Input: part model. Units: mm. Frame: model coordinates. Coordinates: 2 decimals unless noted, no trailing zeros. Order: outer loops, then holes, each group sorted by start corner. A loop starts at its lowest first (then second) coordinate and runs counter-clockwise, first axis right, second up. Notation, with made-up numbers: (-26, -13) -> (29, -13) arc R11 ccw to (29, 4) -> close; hole circle Ø6 at (75, 40.5). An arc over 180 degrees is marked (long way). One line per item, written item: value. Start each with the question number.
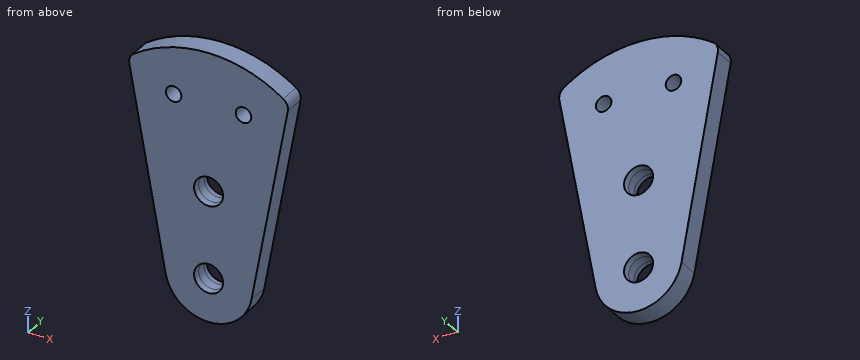
from build123d import *
from OCP.BRepFilletAPI import BRepFilletAPI_MakeChamfer

# Parameters (mm, degrees)
BOSS_EXTRUDE1_DEPTH   = 3.175
F_4_40_TAPPED_HOLE1_D = 2.2606
CUT_EXTRUDE1_REACH    = 37.03
SKETCH3_R             = 1.9812
CHAMFER1_SIZE         = 0.127
CHAMFER1_SIZE2        = 0.903651955


with BuildPart() as part:
    # Sketch2 → Boss-Extrude1 (new body)
    with BuildSketch(Plane(origin=(0, 0, 0), x_dir=(1, 0, 0), z_dir=(0, 1, 0))):
        with BuildLine():
            Line((-6.247852156, 1.134391221), (-11.522869846, -27.918663873))
            ThreePointArc((-11.522869846, -27.918663873), (-11.4270655, -28.816266687), (-10.860710811, -29.519197446))
            ThreePointArc((-10.860710811, -29.519197446), (0, -32.9184), (10.860710811, -29.519197446))
            ThreePointArc((10.860710811, -29.519197446), (11.4270655, -28.816266687), (11.522869846, -27.918663873))
            Line((11.522869846, -27.918663873), (6.247852156, 1.134391221))
            ThreePointArc((6.247852156, 1.134391221), (0, 6.35), (-6.247852156, 1.134391221))
        make_face()
    extrude(amount=BOSS_EXTRUDE1_DEPTH)

    # #4-40 Tapped Hole1 (through all)
    with Locations(Plane(origin=(0, 3.175, 0), x_dir=(1, 0, 0), z_dir=(0, 1, 0))):
        with Locations((-5.08, -25.4), (5.08, -25.4)):
            Hole(F_4_40_TAPPED_HOLE1_D / 2)

    # Sketch3 → Cut-Extrude1 (cut, up to next)
    with BuildSketch(Plane(origin=(0, 3.175, 0), x_dir=(1, 0, 0), z_dir=(0, 1, 0)), mode=Mode.PRIVATE) as cut_extrude1_sk1:
        with Locations(Location((0, 0, 0), (0, 0, 270))):
            Circle(SKETCH3_R)
    cut_extrude1_tool1 = extrude(cut_extrude1_sk1.sketch, amount=-CUT_EXTRUDE1_REACH, mode=Mode.PRIVATE) & part.part
    # Sketch3 → Cut-Extrude1 (cut, up to next)
    with BuildSketch(Plane(origin=(0, 3.175, 0), x_dir=(1, 0, 0), z_dir=(0, 1, 0)), mode=Mode.PRIVATE) as cut_extrude1_sk2:
        with Locations(Location((0, -12.7, 0), (0, 0, 270))):
            Circle(SKETCH3_R)
    cut_extrude1_tool2 = extrude(cut_extrude1_sk2.sketch, amount=-CUT_EXTRUDE1_REACH, mode=Mode.PRIVATE) & part.part
    add(cut_extrude1_tool1.solids().sort_by_distance((0, 3.175, 0))[0], mode=Mode.SUBTRACT)
    add(cut_extrude1_tool2.solids().sort_by_distance((0, 3.175, 12.7))[0], mode=Mode.SUBTRACT)

    # Chamfer1: one chamfer whose edges measure the first distance from different faces: ONE call of the kernel's chamfer builder (chamfer() names one face for all edges)
    chamfer1_edges_1 = [part.edges().sort_by_distance(p)[0] for p in [
        (0, 3.175, -1.9812),
        (0, 3.175, 10.7188),
    ]]
    chamfer1_side_1 = [part.faces().sort_by_distance(p)[0] for p in [
        (0, 3.175, 15.711859533),
    ]]
    chamfer1_edges_2 = [part.edges().sort_by_distance(p)[0] for p in [
        (0, 0, -1.9812),
        (0, 0, 10.7188),
    ]]
    chamfer1_side_2 = [part.faces().sort_by_distance(p)[0] for p in [
        (0, 0, 15.711859533),
    ]]
    chamfer1 = BRepFilletAPI_MakeChamfer(part.part.solid().wrapped)
    for e in chamfer1_edges_1:
        chamfer1.Add(CHAMFER1_SIZE, CHAMFER1_SIZE2, e.wrapped, chamfer1_side_1[0].wrapped)  # the first distance lies on this face
    for e in chamfer1_edges_2:
        chamfer1.Add(CHAMFER1_SIZE, CHAMFER1_SIZE2, e.wrapped, chamfer1_side_2[0].wrapped)  # the first distance lies on this face
    add(Compound.cast(chamfer1.Shape()), mode=Mode.REPLACE)


solid = part.part
1) Section query B-B, the plane y = 1.4. Return the cut outline in (x, z).
2) Pin query (flat end, axial travel): pin 1 Ø4 at (x, z) = (-4, 22) entering from -Y; pin 2 Ø1 at (y, z) = (1, 1) entering from -X; pin 3 Ø1 at (y, z) = (2, 20.5) entering from +X. Return the tip coordinate at first contact, or that it passes through.
3) Ray query, line 1 along Z through (x, y) = (0.75, 0.4); line 2 along X through (y, z) = (2.1, 25); line 3 along Z through (x, y) = (-1, 0.85). Return the intervals inside material, ascending. Write a range as from..to.
4) Section query D-D, the plane x = 5.08. Return the cut outline in (y, z) (3 decimals), plus the area to 3 significant figures.
5) Section query A-A, the plane x = 0. Return the cut outline in (y, z) (3 decimals).
6) Section query C-C, the plane z = 0. Return the cut outline in (x, y) (3 decimals), plus the area to 3 significant figures.
Entries:
1. outline: (-11.52, 27.92) -> (-6.25, -1.13) arc R6.35 ccw to (6.25, -1.13) -> (11.52, 27.92) arc R1.6 ccw to (10.86, 29.52) arc R19.05 ccw to (-10.86, 29.52) arc R1.6 ccw to start; hole circle Ø2.26 at (-5.08, 25.4); hole circle Ø3.96 at (0, 0); hole circle Ø3.96 at (0, 12.7); hole circle Ø2.26 at (5.08, 25.4)
2. pin 1: stops at y = 0
2. pin 2: stops at x = -6.73
2. pin 3: stops at x = 10.27
3. line 1: z = -6.31..-1.91, 1.91..10.79, 14.61..32.9
3. line 2: x = -10.99..-6.14, -4.02..4.02, 6.14..10.99
3. line 3: z = -6.27..-1.72, 1.72..10.98, 14.42..32.89
4. outline: (0, -3.81) -> (3.175, -3.81) -> (3.175, 24.27) -> (0, 24.27) -> close; (0, 26.53) -> (3.175, 26.53) -> (3.175, 32.229) -> (0, 32.229) -> close
4. area: 107 mm2
5. outline: (0, -6.35) -> (3.175, -6.35) -> (3.175, -2.108) -> (2.271, -1.981) -> (0.904, -1.981) -> (0, -2.108) -> close; (0, 2.108) -> (0.904, 1.981) -> (2.271, 1.981) -> (3.175, 2.108) -> (3.175, 10.592) -> (2.271, 10.719) -> (0.904, 10.719) -> (0, 10.592) -> close; (0, 14.808) -> (0.904, 14.681) -> (2.271, 14.681) -> (3.175, 14.808) -> (3.175, 32.918) -> (0, 32.918) -> close
6. outline: (-6.454, 0) -> (-2.108, 0) -> (-1.981, 0.904) -> (-1.981, 2.271) -> (-2.108, 3.175) -> (-6.454, 3.175) -> close; (1.981, 0.904) -> (2.108, 0) -> (6.454, 0) -> (6.454, 3.175) -> (2.108, 3.175) -> (1.981, 2.271) -> close
6. area: 28.2 mm2
